```python
from build123d import *

# Parameters (mm, degrees)
F0_W      = 105
F0_H      = 85
F1_DEPTH  = 2.5
F1_FACE_W = 105
F1_FACE_H = 85
F2_DEPTH  = 2.5
F3_R      = 2.5
F3_R_2    = 0.5
F4_DEPTH  = 25


with BuildPart() as f1:
    # F0 (on Top) → F1 (new body)
    with BuildSketch(Plane.XY):
        Rectangle(F0_W, F0_H)
    extrude(amount=F1_DEPTH)

    # F1_face (on face) → F2 (join)
    with BuildSketch(Plane.XY.offset(2.5)):
        Rectangle(F1_FACE_W, F1_FACE_H)
    extrude(amount=F2_DEPTH)

    # F3 (on face) → F4 (cut)
    with BuildSketch(Plane.XY.offset(5)):
        Circle(F3_R)
        with Locations((-38.084019, -26.250001)):
            Circle(F3_R_2)
        with Locations((-27.540985, -27.110657)):
            Circle(F3_R_2)
        with Locations((-30.768445, -20.225411)):
            Circle(F3_R_2)
        with Locations((-39.375, -20.010246)):
            Circle(F3_R_2)
        with Locations((-33.565577, -34.856558)):
            Circle(F3_R_2)
        with Locations((-39.375, -33.565573)):
            Circle(F3_R_2)
    extrude(amount=-F4_DEPTH, mode=Mode.SUBTRACT)


solid = f1.part
```
The model under review builds one solid part; all positions refer to its coordinate system, in mm. Coordinates: 2 decimals unless noted, no trailing zeros. Write each loop counter-clockwise with the first axis right and the second up, starting at its lowest first coordinate (ties: lowest second). Pieces come first, ordered by that corner, then holes. Notation, with made-up numbers: (10, 12) -> (44, 12) arc R6 cw to (44, 18) -> close; hole circle Ø3 at (74.5, 5.25). An arc over 180 degrees is marked (long way). One line per item, written item: value. Start each with the question number.
Q1. Clearance check with a flat-ended pin moving along its axis: P1, Ø6, axis at x = 0, y = 0, coming from the +Z side. State where the tip first meets the part, or that it passes through.
Q2. To check wall thickness, follow probe 1 along Y at (x, z) = (0, 3); probe 2 along X at (y, z) = (-20, 1.2); probe 3 along X at (y, z) = (-34.5, 2.35). State the ranges of each line that lie inside material, in increasing order.
Q3. Add section A-A, the plane x = 0. Give the boundary of the cut face in (y, z), then the cut area to 3 significant figures.
Q4. The part is to be moulded in two halves that separate along Y. For faces 1 (the face through (-1, 10, 5)), 2 (the face through (-0.54, -2.44, 2.54)), 3 (the face through (-1, -42.5, 2)), 4 (the face through (-1, 42.5, 2)), say which applies: +Y half, -Y half, draft (parallel to the pull), parting line (faces both ways), or undercut.
Q5. Add section B-B, the plane y = 0. Give the boundary of the cut face in (x, z), then the cut area to 3 significant figures.
Response:
1. P1: z = 5
2. probe 1: -42.5 to -2.5, 2.5 to 42.5
2. probe 2: -52.5 to -39.87, -38.88 to -31.21, -30.32 to 52.5
2. probe 3: -52.5 to -33.92, -33.22 to 52.5
3. outline: (-42.5, 0) -> (-2.5, 0) -> (-2.5, 5) -> (-42.5, 5) -> close; (2.5, 0) -> (42.5, 0) -> (42.5, 5) -> (2.5, 5) -> close
3. area: 400 mm²
4. face 1: draft
4. face 2: undercut
4. face 3: -Y half
4. face 4: +Y half
5. outline: (-52.5, 0) -> (-2.5, 0) -> (-2.5, 5) -> (-52.5, 5) -> close; (2.5, 0) -> (52.5, 0) -> (52.5, 5) -> (2.5, 5) -> close
5. area: 500 mm²
